Design review of the part built by this model. Coordinates are the model's own, in mm. Coordinates: 2 decimals unless noted, no trailing zeros. Loops run counter-clockwise (first coordinate to the right, second up) from the corner with the lowest first, then second, coordinate; pieces in that order, holes last. Notation, with made-up numbers: (14, -20) -> (50, -20) arc R23 cw to (50, -11) -> close; hole circle Ø6 at (-13.5, 32.5). An arc over 180 degrees is marked (long way). Use a Markdown table: item, result. Add a question column.
Q1. Take a section at A-A on z = -41. Write out the cut boundary in (x, y).
Q2. For probe 1 along Z at (x, y) = (-0.75, -1.1); probe 2 along X at (y, z) = (-1.05, -35.5); probe 3 along X at (y, z) = (-0.2, -70), list the stretches that pass through material, from the lowest coordinate up.
Q3. Take a section at B-B on x = 1.25. Write out the cut boundary in (y, z).
Q4. Clearance check with a flat-ended pin moving along its axis: pin 1 Ø0.6 at (x, y) = (-3, -0.5) entering from +Z. State where the tip first meets the part, or that it passes through.
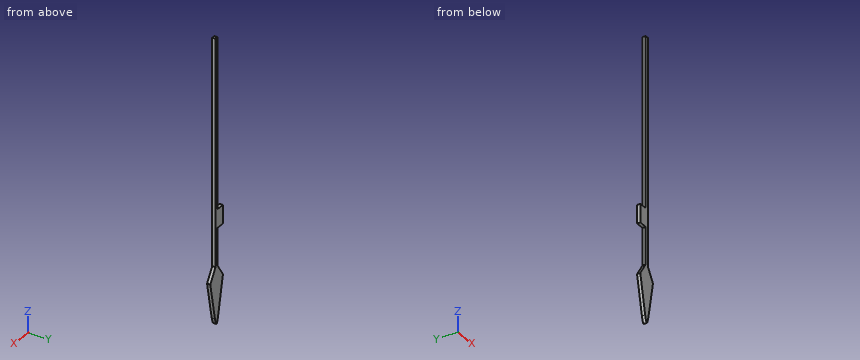
from build123d import *

# Parameters (mm, degrees)
F0_W     = 3.1999936
F0_H     = 7.25000074
F1_DEPTH = 1.27


with BuildPart() as f1:
    # F0 (on Front) → F1 (new body)
    with BuildSketch(Plane.XZ):
        Polygon((-0.065193265, 3.4090982191), (-1.295193345, 3.4090982191), (-1.295193345, -63.3309016509), (-1.295193345, -70.5809023909), (-1.295193345, -85.1709024209), (-0.680193305, -85.1709024209), (-0.065193265, -85.1709024209), align=None)
        with Locations((-2.895190145, -66.9559020209)):
            Rectangle(F0_W, F0_H)
        Polygon((-0.680193305, -104.9110038356), (-0.680193305, -85.1709024209), (-1.295193345, -85.1709024209), (-4.5669513225, -90.2003612126), (-1.6349118244, -104.9110038356), align=None)
        Polygon((3.0674625036, -90.2881598735), (-0.065193265, -85.1709024209), (-0.680193305, -85.1709024209), (-0.680193305, -104.9110038356), (0.2766351171, -105.037851818), align=None)
        with BuildLine():
            Line((0.2766351171, -105.037851818), (-0.680193305, -104.9110038356))
            Line((-0.680193305, -104.9110038356), (-0.680193305, -107.4909024849))
            add(Edge.make_bspline(
                [(-0.680193305, -107.4909024849), (-0.3650057018, -107.493656038), (-0.0441852923, -106.265753928), (0.2766351171, -105.037851818)],
                knots=[0.5054719927, 0.5054719927, 0.5054719927, 0.5054719927, 1, 1, 1, 1], degree=3))
        make_face()
        with BuildLine():
            Line((-0.680193305, -107.4909024849), (-0.680193305, -104.9110038356))
            Line((-0.680193305, -104.9110038356), (-1.6349118244, -104.9110038356))
            add(Edge.make_bspline(
                [(-1.6349118244, -104.9110038356), (-1.3186339428, -106.1995459155), (-1.0023560613, -107.4880879954), (-0.680193305, -107.4909024849)],
                knots=[0, 0, 0, 0, 0.5054719927, 0.5054719927, 0.5054719927, 0.5054719927], degree=3))
        make_face()
    extrude(amount=F1_DEPTH)


solid = f1.part
Answer list:
| question | item | result |
|---|---|---|
| 1 | outline | (-1.3, -1.27) -> (-0.07, -1.27) -> (-0.07, 0) -> (-1.3, 0) -> close |
| 2 | probe 1 | -107.47 to 3.41 |
| 2 | probe 2 | -1.3 to -0.07 |
| 2 | probe 3 | -4.5 to -0.07 |
| 3 | outline | (-1.27, -99.89) -> (0, -99.89) -> (0, -87.32) -> (-1.27, -87.32) -> close |
| 4 | pin 1 | z = -63.33 |
